Input: part model. Units: mm. Frame: model coordinates. Face numbers are marked on the shaded views. A direction names the side the tool comes from. Round coordinates to 2 decimals unless told otherwise and drop trailing zeros. Loops run counter-clockwise (first coordinate to the right, second up) from the corner with the lowest first, then second, coordinate; pieces in that order, holes last.
1) Access query for the marked faces 3, 4, 5, 6 and 7. Directions: +Z, -Z, +X, -X, +Y, -Y. A direction counts if a zero-diameter tool reaches every point of the face in a straight line with its end or side. Return the directions, or none.
2) First-contact query: pin 1 (1 mm diameter, centred on y = -16.5, z = 2.5, fed in from +X); pin 2 (4 mm diameter, centred on x = 14.5, z = 4, fed in from +Y); pin 3 (5 mm diameter, centred on x = -28, z = -2, fed in from -Y). Flat tips, straight axial feed; report the tip coordinate or a pass-through.
3) Section C-C, the plane y = -3.5. Return loops of the section in (x, z).
4) Section A-A, the plane z = 0.25. Return loops of the section in (x, y).
5) Section B-B, the plane y = -70. Return loops of the section in (x, z), and give its area (3 significant figures).
6) Ray query, line 1 along X through (y, z) = (2.5, -1); line 2 along X through (y, z) = (-77, -2.75); line 3 along Z through (x, y) = (25.5, -45). Return the intervals inside material, ascending.
7) Draft query along Y for the marked faces 1 and 2. Return one class per face: pulls with the +Y half, pulls with the -Y half, needs draft (parallel to the pull), parting line crosses it, or undercut.
8) Section D-D, the plane x = -41. Return loops of the section in (y, z), and give its area (3 significant figures).
from build123d import *

# Parameters (mm, degrees)
SKETCH1_R             = 30
SKETCH1_R_2           = 5
SKETCH1_R_3           = 8
BOSS_EXTRUDE1_DEPTH   = 5
SKETCH1_R_4           = 15
SKETCH1_R_5           = 10
BOSS_EXTRUDE1_2_DEPTH = 5
BOSS_EXTRUDE1_3_DEPTH = 5
BOSS_EXTRUDE2_DEPTH   = 2.5


with BuildPart() as part:
    # Sketch1 → Boss-Extrude1 (new, symmetric)
    with BuildSketch(Plane.XY):
        Circle(SKETCH1_R)
        with Locations((-20, 0)):
            Circle(SKETCH1_R_2, mode=Mode.SUBTRACT)
        with Locations((0, -20)):
            Circle(SKETCH1_R_2, mode=Mode.SUBTRACT)
        with Locations((20, 0)):
            Circle(SKETCH1_R_2, mode=Mode.SUBTRACT)
        with Locations((0, 20)):
            Circle(SKETCH1_R_2, mode=Mode.SUBTRACT)
        Circle(SKETCH1_R_3, mode=Mode.SUBTRACT)
    extrude(amount=BOSS_EXTRUDE1_DEPTH, both=True)



with BuildPart() as body_2:
    # Sketch1 → Boss-Extrude1 2 (new, symmetric)
    with BuildSketch(Plane.XY):
        with Locations((-40, -70)):
            Circle(SKETCH1_R_4)
        with Locations((-40, -70)):
            Circle(SKETCH1_R_5, mode=Mode.SUBTRACT)
    extrude(amount=BOSS_EXTRUDE1_2_DEPTH, both=True)


with BuildPart() as body_3:
    # Sketch1 → Boss-Extrude1 3 (new, symmetric)
    with BuildSketch(Plane.XY):
        with Locations((40, -70)):
            Circle(SKETCH1_R_4)
        with Locations((40, -70)):
            Circle(SKETCH1_R_5, mode=Mode.SUBTRACT)
    extrude(amount=BOSS_EXTRUDE1_3_DEPTH, both=True)


with BuildPart() as part_1:
    add(part.part)

    add(body_2.part)  # Boss-Extrude2 merges body 2

    add(body_3.part)  # Boss-Extrude2 merges body 3
    # Sketch1_3 → Boss-Extrude2 (add, symmetric)
    with BuildSketch(Plane.XY):
        with BuildLine():
            Line((-28.361736144, 9.778134939), (-54.180868072, -65.11093253))
            ThreePointArc((-54.180868072, -65.11093253), (-37.521393646, -55.206200267), (-25, -70))
            ThreePointArc((-25, -70), (-26.866074463, -77.245688373), (-32, -82.68857754))
            ThreePointArc((-32, -82.68857754), (0, -73.442887702), (32, -82.68857754))
            ThreePointArc((32, -82.68857754), (30.683660399, -58.24390301), (54.180868072, -65.11093253))
            Line((54.180868072, -65.11093253), (28.361736144, 9.778134939))
            ThreePointArc((28.361736144, 9.778134939), (29.587599466, 4.957212709), (30, 0))
            ThreePointArc((30, 0), (-4.957212709, -29.587599466), (-28.361736144, 9.778134939))
        make_face()
    extrude(amount=BOSS_EXTRUDE2_DEPTH, both=True)


solid = part_1.part
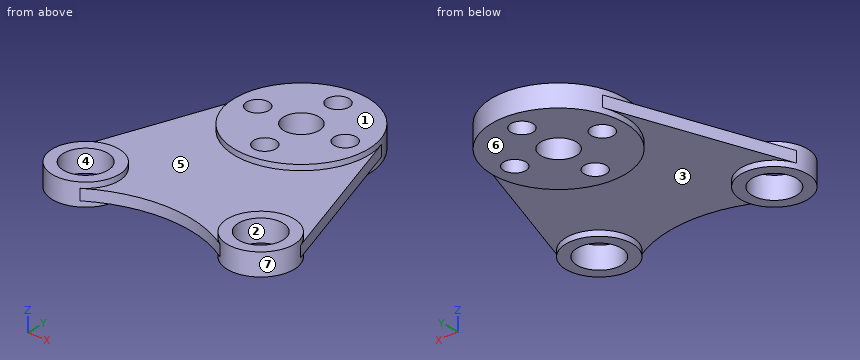
Final values:
1. face 3: -Z
1. face 4: +Z, -Z
1. face 5: +Z
1. face 6: -Z, +X, -X, +Y, -Y
1. face 7: none
2. pin 1: stops at x = 37.59
2. pin 2: stops at y = 27.27
2. pin 3: stops at y = -81.77
3. outline: (-32.94, -2.5) - (-29.8, -2.5) - (-29.8, -5) - (-23.57, -5) - (-23.57, 5) - (-29.8, 5) - (-29.8, 2.5) - (-32.94, 2.5) - close; (-16.43, -5) - (-7.19, -5) - (-7.19, 5) - (-16.43, 5) - close; (7.19, -5) - (16.43, -5) - (16.43, 5) - (7.19, 5) - close; (23.57, -5) - (29.8, -5) - (29.8, -2.5) - (32.94, -2.5) - (32.94, 2.5) - (29.8, 2.5) - (29.8, 5) - (23.57, 5) - close
4. outline: (-54.18, -65.11) arc R15 ccw to (-32, -82.69) arc R60 cw to (32, -82.69) arc R15 ccw to (54.18, -65.11) - (28.36, 9.78) arc R30 ccw to (-28.36, 9.78) - close; hole circle Ø20 at (-40, -70); hole circle Ø10 at (-20, 0); hole circle Ø16 at (0, 0); hole circle Ø10 at (0, -20); hole circle Ø10 at (0, 20); hole circle Ø10 at (20, 0); hole circle Ø20 at (40, -70)
5. outline: (-55, -5) - (-50, -5) - (-50, 5) - (-55, 5) - close; (-30, -5) - (-25, -5) - (-25, -2.5) - (25, -2.5) - (25, -5) - (30, -5) - (30, 5) - (25, 5) - (25, 2.5) - (-25, 2.5) - (-25, 5) - (-30, 5) - close; (50, -5) - (55, -5) - (55, 5) - (50, 5) - close
5. area: 450 mm2
6. line 1: x = -30.87 to -24.33, -15.67 to -7.6, 7.6 to 15.67, 24.33 to 30.87
6. line 2: x = -53.27 to -47.14, -32.86 to -26.73, 26.73 to 32.86, 47.14 to 53.27
6. line 3: z = -2.5 to 2.5
7. face 1: needs draft
7. face 2: undercut
8. outline: (-84.97, -5) - (-79.95, -5) - (-79.95, 5) - (-84.97, 5) - close; (-60.05, -5) - (-55.03, -5) - (-55.03, -2.5) - (-26.88, -2.5) - (-26.88, 2.5) - (-55.03, 2.5) - (-55.03, 5) - (-60.05, 5) - close
8. area: 241 mm2
